from build123d import *

# Parameters (mm, degrees)
SKETCH1_W           = 2.5
SKETCH1_H           = 3
BOSS_EXTRUDE1_DEPTH = 1
SKETCH2_W           = 1
SKETCH2_H           = 3
BOSS_EXTRUDE2_DEPTH = 3
SKETCH3_W           = 0.5
SKETCH3_H           = 3
BOSS_EXTRUDE3_DEPTH = 3
SKETCH4_W           = 3
SKETCH4_H           = 0.5
BOSS_EXTRUDE4_DEPTH = 3
SKETCH5_W           = 3
SKETCH5_H           = 0.5
BOSS_EXTRUDE5_DEPTH = 2.5
SKETCH8_W           = 2.5
SKETCH8_H           = 3
BOSS_EXTRUDE6_DEPTH = 4
FILLET1_R           = 0.5


with BuildPart() as part:
    # Sketch1 → Boss-Extrude1 (new body)
    with BuildSketch(Plane(origin=(0, 0, 0), x_dir=(1, 0, 0), z_dir=(0, 1, 0))):
        Rectangle(SKETCH1_W, SKETCH1_H)
    extrude(amount=BOSS_EXTRUDE1_DEPTH)

    # Sketch2 → Boss-Extrude2 (add)
    with BuildSketch(Plane.XZ):
        with Locations((0.75, 0)):
            Rectangle(SKETCH2_W, SKETCH2_H)
    extrude(amount=BOSS_EXTRUDE2_DEPTH)

    # Sketch3 → Boss-Extrude3 (add)
    with BuildSketch(Plane.XZ):
        with Locations((-1, 0)):
            Rectangle(SKETCH3_W, SKETCH3_H)
    extrude(amount=BOSS_EXTRUDE3_DEPTH)

    # Sketch4 → Boss-Extrude4 (add)
    with BuildSketch(Plane(origin=(1.25, 0, 0), x_dir=(0, 0, -1), z_dir=(1, 0, 0))):
        with Locations((0, -0.25)):
            Rectangle(SKETCH4_W, SKETCH4_H)
    extrude(amount=BOSS_EXTRUDE4_DEPTH)

    # Sketch5 → Boss-Extrude5 (add)
    with BuildSketch(Plane.ZY.offset(1.25)):
        with Locations((0, -0.25)):
            Rectangle(SKETCH5_W, SKETCH5_H)
    extrude(amount=BOSS_EXTRUDE5_DEPTH)

    # Sketch8 → Boss-Extrude6 (add)
    with BuildSketch(Plane(origin=(0, 1, 0), x_dir=(1, 0, 0), z_dir=(0, 1, 0))):
        Rectangle(SKETCH8_W, SKETCH8_H)
    extrude(amount=BOSS_EXTRUDE6_DEPTH)

    # Fillet1
    fillet1_edges = [part.edges().sort_by_distance(p)[0] for p in [
        (1.25, 2.5, 1.5),
        (-1.25, 2.5, 1.5),
        (-1.25, 2.5, -1.5),
        (1.25, 2.5, -1.5),
    ]]
    fillet(fillet1_edges, radius=FILLET1_R - 0.0001)  # a hair under: the kernel refuses the full size


solid = part.part
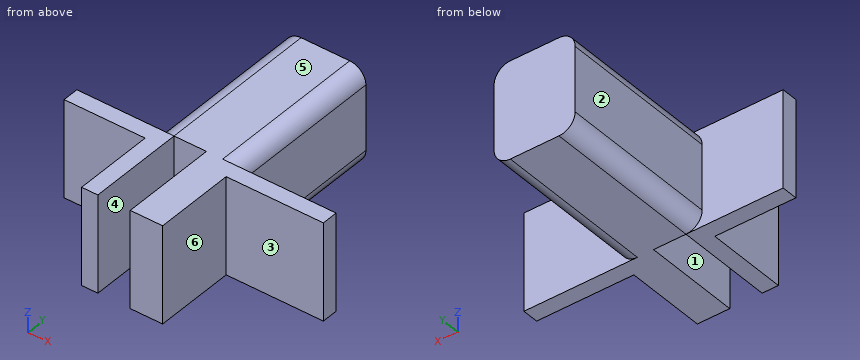
Geometry: final body of the model. Coordinates: model frame, mm. Face numbers are marked on the shaded views. A direction names the side the tool comes from. Round coordinates to 2 decimals unless told otherwise and drop trailing zeros. Order: outer loops, then holes, each group sorted by start corner. A loop starts at its lowest first (then second) coordinate and runs counter-clockwise, first axis right, second up.
Q1. Material intervals for probe 1 along X at (y, z) = (-0.75, -0.35); probe 2 along X at (y, z) = (-0.25, -0.45); probe 3 along Y at (x, z) = (3, 1.2), sorted ascending.
Result sheet:
probe 1: x = -1.25 to -0.75, 0.25 to 1.25
probe 2: x = -3.75 to -0.75, 0.25 to 4.25
probe 3: y = -0.5 to 0
Q2. Mould query, pull axis X, two halves, no side actions, for the marked faces 4, 5 and 6. Classes: released by +X, released by -X, zero draft, split by the parting line, or undercut.
Result sheet:
face 4: undercut
face 5: zero draft
face 6: released by +X
Q3. Access query for the marked faces 1, 2 and 3. Directions: +Z, -Z, +X, -X, +Y, -Y. A direction counts if a zero-diameter tool reaches every point of the face in a straight line with its end or side. Return the directions, or none.
Result sheet:
face 1: +Z, -Z, -Y
face 2: +Z, -Z, -X, +Y
face 3: +Z, -Z, +X, -Y
Q4. Section C-C, the plane x = 1. Output: boundary loops of the cut face in (y, z), and give its area (3 significant figures).
Result sheet:
outline: (-3, -1.5) - (0, -1.5) - (0, -1.43) - (5, -1.43) - (5, 1.43) - (0, 1.43) - (0, 1.5) - (-3, 1.5) - close
area: 23.3 mm2
Q5. Section B-B, the plane z = 0.7. Output: boundary loops of the cut face in (x, y), and give its area (4 significant figures).
Result sheet:
outline: (-3.75, -0.5) - (-1.25, -0.5) - (-1.25, -3) - (-0.75, -3) - (-0.75, 0) - (0.25, 0) - (0.25, -3) - (1.25, -3) - (1.25, -0.5) - (4.25, -0.5) - (4.25, 0) - (1.25, 0) - (1.25, 5) - (-1.25, 5) - (-1.25, 0) - (-3.75, 0) - close
area: 19.75 mm2
Q6. Section D-D, the plane y = 2.5. Output: boundary loops of the cut face in (x, z).
Result sheet:
outline: (-1.25, -1) arc R0.5 ccw to (-0.75, -1.5) - (0.75, -1.5) arc R0.5 ccw to (1.25, -1) - (1.25, 1) arc R0.5 ccw to (0.75, 1.5) - (-0.75, 1.5) arc R0.5 ccw to (-1.25, 1) - close
Q7. Pin query (flat end, axial travel): pin 1 (0.9 mm diameter, centred on y = -1.5, z = 0, fed in from +X); pin 2 (1 mm diameter, centred on x = -1.5, y = 1.5, fed in from -Z); pin 3 (1.5 mm diameter, centred on y = -1.5, z = -0.5, fed in from -X). Return the tip coordinate at first contact, or that it passes through.
Result sheet:
pin 1: stops at x = 1.25
pin 2: stops at z = -1.43
pin 3: stops at x = -1.25
Q8. Section A-A, the plane y = -1. Output: boundary loops of the cut face in (x, z).
Result sheet:
outline: (-1.25, -1.5) - (-0.75, -1.5) - (-0.75, 1.5) - (-1.25, 1.5) - close; (0.25, -1.5) - (1.25, -1.5) - (1.25, 1.5) - (0.25, 1.5) - close
